Design review of the part built by this model. Coordinates are the model's own, in mm. A direction names the side the tool comes from. Round coordinates to 2 decimals unless told otherwise and drop trailing zeros. Loops run counter-clockwise (first coordinate to the right, second up) from the corner with the lowest first, then second, coordinate; pieces in that order, holes last. Notation, with made-up numbers: M 17,66.5 L 46,66.5 A22 cw 46,95.5 Z; hole C 72,-29 d7. An arc over 180 degrees is marked long. One line per item, written item: value. Start each with the question number.
Item 1: Mouldability with a two-part tool opening along Z and no side actions: class faces 1 (the flat face through (-8, 11.59, 20)), 2 (the cylindrical face through (-9.1, 10.9, 5.7)), 3 (the flat face through (-8, 11, 0)) as released by +Z, released by -Z, zero draft, split by the parting line, or undercut.
Item 2: We need section C-C (y = 11.05). Write out the cut boundary in (x, z).
Item 3: We need section A-A (z = 5). Write out the cut boundary in (x, y).
Item 4: We need section B-B (x = -7). Write out the cut boundary in (y, z).
Item 5: For line 1 along X through (y, z) = (10.7, 5); line 2 along Z through (x, y) = (-7.75, 10.4); line 3 along X through (y, z) = (11.1, 37), list the stretches that pass through material, from the lowest coordinate up.
Item 6: Clearance check with a flat-ended pin moving along its axis: pin 1 (2.5 mm diameter, centred on x = -7.77, z = 5, fed in from +Y). State where the tip first meets the part, or that it passes through.
Item 7: We need section D-D (z = 33.5). Write out the cut boundary in (x, y).
Item 8: For faces 4 (the flat face through (-11.759, 10.851, 29.028)), 5 (the flat face through (-2.773, 11, 16)), list the 3-axis set-ups (+Z, -Z, +X, -X, +Y, -Y) from which the entire face can be reached by the end or side of a thin tool; tool diameter is ignored.
from build123d import *

# Parameters (mm, degrees)
ESQUISSE1_W      = 10
ESQUISSE1_H      = 1.5
EXTRUSION1_DEPTH = 40
ESQUISSE2_R      = 1
ESQUISSE2_R_2    = 1.5
EXTRUSION2_DEPTH = 50


with BuildPart() as part:
    # Esquisse1 → Extrusion1 (new body)
    with BuildSketch(Plane.XY):
        with Locations((-7.772581117, 10.840421053)):
            Rectangle(ESQUISSE1_W, ESQUISSE1_H)
    extrude(amount=EXTRUSION1_DEPTH)

    # Esquisse2 → Extrusion2 (cut)
    with BuildSketch(Plane(origin=(0, 11.590421053, 0), x_dir=(-1, 0, 0), z_dir=(0, 1, 0))):
        with Locations(Location((9.772581117, 37, 0), (0, 0, 90))):
            Circle(ESQUISSE2_R)
        with Locations(Location((7.772581117, 5, 0), (0, 0, 90))):
            Circle(ESQUISSE2_R_2)
        Polygon((12.772581117, 35), (10.772581117, 31), (12.772581117, 27), align=None)
        Polygon((5.772581117, 40), (2.772581117, 40), (2.772581117, 33), align=None)
    extrude(amount=-EXTRUSION2_DEPTH, mode=Mode.SUBTRACT)


solid = part.part
A:
1. face 1: zero draft
1. face 2: undercut
1. face 3: released by -Z
2. outline: M -12.77,0 L -2.77,0 L -2.77,33 L -5.77,40 L -12.77,40 L -12.77,35 L -10.77,31 L -12.77,27 Z; hole C -9.77,37 d2; hole C -7.77,5 d3
3. outline: M -12.77,10.09 L -9.27,10.09 L -9.27,11.59 L -12.77,11.59 Z; M -6.27,10.09 L -2.77,10.09 L -2.77,11.59 L -6.27,11.59 Z
4. outline: M 10.09,0 L 11.59,0 L 11.59,3.71 L 10.09,3.71 Z; M 10.09,6.29 L 11.59,6.29 L 11.59,40 L 10.09,40 Z
5. line 1: -12.77 to -9.27, -6.27 to -2.77
5. line 2: 0 to 3.5, 6.5 to 40
5. line 3: -12.77 to -10.77, -8.77 to -4.49
6. pin 1: through
7. outline: M -12.02,10.09 L -2.99,10.09 L -2.99,11.59 L -12.02,11.59 Z
8. face 4: -X, +Y, -Y
8. face 5: +Z, -Z, +X, +Y, -Y
